```python
from build123d import *

# Parameters (mm, degrees)
SCHNITT_LINEAR_AUSTRAGEN1_DEPTH = 1.8
FASE1_SIZE                      = 0.2
VERRUNDUNG1_R                   = 0.2
VERRUNDUNG2_R                   = 0.1


with BuildPart() as part:
    # Skizze1 → Rotation1 (revolve)
    with BuildSketch(Plane(origin=(0, 0, 0), x_dir=(0, 0, -1), z_dir=(1, 0, 0))):
        Polygon((-3, 0), (-3, 2.75), (0, 2.75), (0, 1.465), (16, 1.465), (16, 0), align=None)
    revolve(axis=Axis((0, 0, 21.919879518), (0, 0, -1)))

    # Skizze2 → Schnitt-Linear austragen1 (cut)
    with BuildSketch(Plane.XY.offset(3)):
        Polygon((1.25, -0.721687836), (1.25, 0.721687836), (0, 1.443375673), (-1.25, 0.721687836), (-1.25, -0.721687836), (0, -1.443375673), align=None)
    extrude(amount=-SCHNITT_LINEAR_AUSTRAGEN1_DEPTH, mode=Mode.SUBTRACT)

    # Fase1
    fase1_edges = [part.edges().sort_by_distance(p)[0] for p in [
        (0, -1.465, -16),
        (0, -2.75, 0),
        (0, -2.75, 3),
    ]]
    chamfer(fase1_edges, length=FASE1_SIZE)

    # Verrundung1
    verrundung1_edges = [part.edges().sort_by_distance(p)[0] for p in [
        (0.625, -1.082531755, 1.2),
        (1.25, -0.721687836, 2.1),
        (-0.625, -1.082531755, 1.2),
        (0, -1.443375673, 2.1),
        (-1.25, 0, 1.2),
        (-1.25, -0.721687836, 2.1),
        (-0.625, 1.082531755, 1.2),
        (-1.25, 0.721687836, 2.1),
        (0.625, 1.082531755, 1.2),
        (0, 1.443375673, 2.1),
        (1.25, 0, 1.2),
        (1.25, 0.721687836, 2.1),
        (0, -1.465, 0),
    ]]
    fillet(verrundung1_edges, radius=VERRUNDUNG1_R)

    # Verrundung2
    verrundung2_edges = [part.edges().sort_by_distance(p)[0] for p in [
        (-0.625, -1.082531755, 3),
        (-1.25, 0, 3),
        (-0.625, 1.082531755, 3),
        (0.625, 1.082531755, 3),
        (1.25, 0, 3),
        (0.625, -1.082531755, 3),
        (-1.223205081, -0.706217783, 3),
        (0, -1.412435565, 3),
        (1.223205081, -0.706217783, 3),
        (1.223205081, 0.706217783, 3),
        (0, 1.412435565, 3),
        (-1.223205081, 0.706217783, 3),
    ]]
    fillet(verrundung2_edges, radius=VERRUNDUNG2_R)


solid = part.part
```
Geometry check sheet. Reference: the model listing, model coordinates, mm. A direction names the side the tool comes from. Coordinates: 2 decimals unless noted, no trailing zeros. Write each loop counter-clockwise with the first axis right and the second up, starting at its lowest first coordinate (ties: lowest second). Pieces come first, ordered by that corner, then holes. Notation, with made-up numbers: M 80,32 L 97,32 A21 cw 97,44 Z; hole C 39,61.5 d6. An arc over 180 degrees is marked long. One line per item, written item: value. Start each with the question number.
(1) Sectioned sample at A-A, the plane y = 0. Enter the section's corners in (x, z) (3 decimals), and give its area (3 significant figures).
(2) Release check for a two-part mould opening along X. For faces 4 (the face through (0.63, 1.08, 2.16)), 5 (the face through (-1.43, -0.32, -8.11)), 6 (the face through (-1.1, -1.1, 3)) record: released by +X, released by -X, zero draft, split by the parting line, or undercut.
(3) Depth check by flat-ended pin: pin 1 (3 mm diameter, centred on x = 0, z = -2.5, fed in from +Y) (3 decimals); pin 2 (0.6 mm diameter, centred on x = -0.5, y = 0, fed in from +Z); pin 3 (1 mm diameter, centred on x = -1, z = -6, fed in from -Y). Enter the tip coordinate at first touch or a pass-through.
(4) Tool access check on faces 1 (the face through (-1, 2, 0)), 2 (the face through (0, 0, 1.2)), 3 (the face through (-2.685, -0.596, 1.482)). Record the directions out of +Z, -Z, +X, -X, +Y, -Y that give a thin tool (end or side, any length) a straight path to the whole face; none if there is none.
(5) Sectioned sample at B-B, the plane z = -7.5. Enter the section's corners in (x, y) (3 decimals).
(6) Scan lines: line 1 along Z through (x, y) = (-0.5, 0.45); line 2 along Z through (x, y) = (-1.15, 2); line 3 along X through (y, z) = (-0.3, 1.5). Record each from-to range of solid material in increasing order. Write a range as [from, to].
(7) Sectioned sample at C-C, the plane z = 1. Enter the section's corners in (x, y).
Filled sheet:
1. outline: M -2.75,0.2 L -2.55,0 L -1.665,0 A0.2 cw -1.465,-0.2 L -1.465,-15.8 L -1.265,-16 L 1.265,-16 L 1.465,-15.8 L 1.465,-0.2 A0.2 cw 1.665,0 L 2.55,0 L 2.75,0.2 L 2.75,2.8 L 2.55,3 L 1.35,3 A0.1 ccw 1.25,2.9 L 1.25,1.4 A0.2 cw 1.05,1.2 L -1.05,1.2 A0.2 cw -1.25,1.4 L -1.25,2.9 A0.1 ccw -1.35,3 L -2.55,3 L -2.75,2.8 Z
1. area: 58.8 mm²
2. face 4: undercut
2. face 5: split by the parting line
2. face 6: zero draft
3. pin 1: y = 1.465
3. pin 2: z = 1.2
3. pin 3: y = -1.38
4. face 1: -Z
4. face 2: +Z
4. face 3: +Z, -Z
5. outline: C 0,0 d2.93
6. line 1: [-16, 1.2]
6. line 2: [0, 3]
6. line 3: [-2.73, -1.25], [1.25, 2.73]
7. outline: C 0,0 d5.5
